Can you work these out from the model? Positions are in its coordinate system, mm. Face numbers are marked on the shaded views. Round coordinates to 2 decimals unless told otherwise and drop trailing zeros. Write each loop counter-clockwise with the first axis right and the second up, starting at its lowest first coordinate (ties: lowest second). Pieces come first, ordered by that corner, then holes. Notation, with made-up numbers: (76.5, 19.5) - (109.5, 19.5) arc R19 cw to (109.5, 30.5) - close; hole circle Ø7 at (59.25, 65). An arc over 180 degrees is marked (long way). One line per item, written item: value. Start each with the question number.
(1) I want a section at A-A on y = 7.5. List the corners of the cut face in (x, z) for me, plus the area to 3 significant figures.
(2) If I drill on L1, parallel to X at y = 5, z = 0; L2, parallel to Z at x = -6.5, y = 1.5; L3, parallel to Z at x = -6, y = 8.25, over which ranges is the centre line in solid material (lowest first)? Write a range as from..to.
(3) Thinking about a two-plate mould opening in Z: for the marked faces 1, 2 and 3, which applies, +Z half, -Z half, draft (parallel to the pull), parting line (faces both ways), or undercut?
(4) I'm going to push flat-ended pins straight in: pin 1 Ø1 at (x, y) = (4.5, 1) entering from +Z; pin 2 Ø1.5 at (x, y) = (-1.5, 7) entering from -Z; pin 3 Ø2 at (x, y) = (7.5, 1) entering from +Z. Where does each tip first touch, or does it pass through?
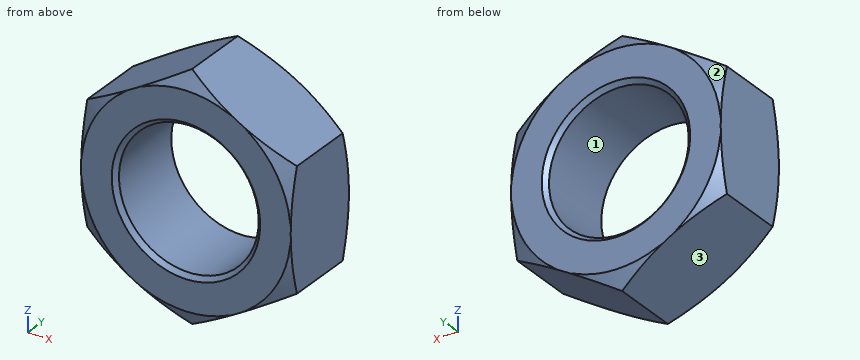
Autodesk Inventor part; units mm, degrees
ref_plane "YZ Plane" through (0, 0, 0) normal (1, 0, 0) x (0, 1, 0)
ref_plane "XZ Plane" through (0, 0, 0) normal (0, 1, 0) x (-1, 0, 0)
ref_plane "XY Plane" through (0, 0, 0) normal (0, 0, 1) x (1, 0, 0)
sketch "Sketch1" plane through (0, 0, 0) normal (0, 1, 0) x (-1, 0, 0)
  line L0 (12, -6.9282) -> (0, -13.8564)
  line L1 (0, -13.8564) -> (-12, -6.9282)
  line L2 (-12, -6.9282) -> (-12, 6.9282)
  line L3 (-12, 6.9282) -> (0, 13.8564)
  line L4 (0, 13.8564) -> (12, 6.9282)
  line L5 (12, 6.9282) -> (12, -6.9282)
  point P0 (0, 0)
  point P1 (0, 0)
  point P2 (-12, 0)
  point P3 (12, 0)
  dimension "d0" = 24
extrude "Extrusion1" add sketch "Sketch1" along normal blind 10
sketch "Sketch2" plane through (0, 10, 0) normal (0, 1, 0) x (1, 0, 0)
  circle A0 centre (0, 0) radius 12
extrude "Extrusion2" cut sketch "Sketch2" against normal blind 10 draft 60 keep common part
sketch "Sketch4" plane through (0, 0, 0) normal (0, -1, 0) x (1, 0, 0)
  circle A0 centre (0, 0) radius 12
extrude "Extrusion4" cut sketch "Sketch4" against normal blind 60 draft 60 keep common part
sketch "Sketch5" plane through (0, 10, 0) normal (0, 1, 0) x (1, 0, 0)
  point P0 (0, 0)
  point P1 (0, 0)
hole "Hole1" at (0, 10, 0) direction (0, -1, 0) diameter 16 end through all
thread "Thread2"
chamfer "Chamfer2" distance 0.5 angle 45 2 edges at (0, 10, -8) (0, 0, -8)
properties part number "csavar" material "Steel, Alloy"
Established:
1. outline: (-12, -6.93) - (0, -13.86) - (12, -6.93) - (12, 6.93) - (0, 13.86) - (-12, 6.93) - close; hole circle Ø16 at (0, 0)
1. area: 298 mm2
2. L1: -12..-8, 8..12
2. L2: -10.1..-4.66, 4.66..10.1
2. L3: -10.39..-5.29, 5.29..10.39
3. face 1: undercut
3. face 2: +Z half
3. face 3: -Z half
4. pin 1: z = 11.55
4. pin 2: z = -13.42
4. pin 3: z = 10.1
